from build123d import *
from build123d.topology import SkipClean

# Parameters (mm, degrees)
BOSS_EXTRUDE1_DEPTH     = 2
SKETCH2_R               = 1.9
BOSS_EXTRUDE2_DEPTH     = 2
CUT_EXTRUDE1_REACH      = 24.481
SKETCH4_R               = 4
BOSS_EXTRUDE3_REACH     = 24.481
BOSS_EXTRUDE4_DEPTH     = 2
BOSS_EXTRUDE5_DEPTH     = 2
CUT_EXTRUDE2_DEPTH      = 0.3
REVOLVE1_ANGLE          = 180
CUT_EXTRUDE3_DEPTH      = 24.576202563
CUT_EXTRUDE3_DEPTH_BACK = 24.576202563


with BuildPart() as part:
    # Sketch1 → Boss-Extrude1 (new body)
    with BuildSketch(Plane.XY):
        with BuildLine():
            Line((-4, -10), (4, -10))
            ThreePointArc((4, -10), (5.414213562, -9.414213562), (6, -8))
            Line((6, -8), (6, 6))
            Line((6, 6), (3.305891799, 20.36857707))
            ThreePointArc((3.305891799, 20.36857707), (2.6174191, 21.539018216), (1.340147425, 22))
            Line((1.340147425, 22), (-1.340147425, 22))
            ThreePointArc((-1.340147425, 22), (-2.6174191, 21.539018216), (-3.305891799, 20.36857707))
            Line((-3.305891799, 20.36857707), (-6, 6))
            Line((-6, 6), (-6, -8))
            ThreePointArc((-6, -8), (-5.414213562, -9.414213562), (-4, -10))
        make_face()
    extrude(amount=BOSS_EXTRUDE1_DEPTH)

    # Sketch2 → Boss-Extrude2 (add)
    with BuildSketch(Plane(origin=(0, 1.005401315, 5.701914197), x_dir=(-1, 0, 0), z_dir=(0, 0.1736481776669307, 0.984807753012208))):
        with BuildLine():
            Line((-3.6, -1.961550163), (-3.6, -5.561550163))
            Line((-3.6, -5.561550163), (-6, -5.561550163))
            Line((-6, -5.561550163), (-3.305891799, -19.711836261))
            add(Edge.make_bspline(
                [(-3.305891799, -19.711836261), (-3, -21.318474211), (-1.340147425, -21.318474211)],
                knots=[3.326940604, 3.326940604, 3.326940604, 4.71238898, 4.71238898, 4.71238898], degree=2, weights=[1, 0.769509108, 1]))
            Line((-1.340147425, -21.318474211), (1.340147425, -21.318474211))
            add(Edge.make_bspline(
                [(1.340147425, -21.318474211), (3, -21.318474211), (3.305891799, -19.711836261)],
                knots=[4.71238898, 4.71238898, 4.71238898, 6.097837357, 6.097837357, 6.097837357], degree=2, weights=[1, 0.769509108, 1]))
            Line((3.305891799, -19.711836261), (6, -5.561550163))
            Line((6, -5.561550163), (3.6, -5.561550163))
            Line((3.6, -5.561550163), (3.6, -1.961550163))
            ThreePointArc((3.6, -1.961550163), (0, 1.638449837), (-3.6, -1.961550163))
        make_face()
        with Locations(Location((0, -1.961550163, 0), (0, 0, 90))):
            Circle(SKETCH2_R, mode=Mode.SUBTRACT)
    extrude(amount=-BOSS_EXTRUDE2_DEPTH)

    # Cut-Extrude1: up to this plane
    cut_extrude1_end = Plane(origin=(1.340147425, 20, 0), z_dir=(0, 0, 1))
    # Sketch4 → Cut-Extrude1 (cut, up to the surface)
    with BuildSketch(Plane(origin=(0, 0.658104959, 3.732298691), x_dir=(-1, 0, 0), z_dir=(0, -0.1736481776669307, -0.9848077530122081)), mode=Mode.PRIVATE) as cut_extrude1_sk1:
        with Locations(Location((0, 1.961550163, 0), (0, 0, 90))):
            Circle(SKETCH4_R)
    cut_extrude1_tool1 = split(extrude(cut_extrude1_sk1.sketch, amount=CUT_EXTRUDE1_REACH, mode=Mode.PRIVATE), bisect_by=cut_extrude1_end, keep=Keep.BOTH, mode=Mode.PRIVATE)
    add(cut_extrude1_tool1.solids().sort_by_distance((0, 2.589855, 3.391679))[0], mode=Mode.SUBTRACT)

    # Sketch5 → Boss-Extrude3 (add, up to next)
    with BuildSketch(Plane(origin=(0, 0.658104959, 3.732298691), x_dir=(-1, 0, 0), z_dir=(0, -0.1736481776669307, -0.9848077530122081)), mode=Mode.PRIVATE) as boss_extrude3_sk1:
        with BuildLine():
            Line((-6, 5.561550163), (-4, 5.561550163))
            ThreePointArc((-4, 5.561550163), (0, 7.342999782), (4, 5.561550163))
            Line((4, 5.561550163), (6, 5.561550163))
            Line((6, 5.561550163), (5.159538931, 9.975910572))
            Line((5.159538931, 9.975910572), (-5.159538931, 9.975910572))
            Line((-5.159538931, 9.975910572), (-6, 5.561550163))
        make_face()
    boss_extrude3_tool1 = extrude(boss_extrude3_sk1.sketch, amount=BOSS_EXTRUDE3_REACH, mode=Mode.PRIVATE) - part.part
    add(boss_extrude3_tool1.solids().sort_by_distance((0, 8.606511, 2.33078))[0])

    # Sketch6 → Boss-Extrude4 (add)
    with BuildSketch(Plane(origin=(6, 0, 0), x_dir=(0, 0, -1), z_dir=(1, 0, 0))):
        Polygon((-4.736161147, 6.482459034), (-2, 6), (-2, -8), align=None)
    extrude(amount=-BOSS_EXTRUDE4_DEPTH)

    # Sketch7 → Boss-Extrude5 (add)
    with BuildSketch(Plane.ZY.offset(6)):
        Polygon((2, 6), (4.736161147, 6.482459034), (2, -8), align=None)
    extrude(amount=-BOSS_EXTRUDE5_DEPTH)

    # Sketch8 → Cut-Extrude2 (cut)
    with BuildSketch(Plane(origin=(0, 0, 0), x_dir=(-1, 0, 0), z_dir=(0, 0, -1))):
        with BuildLine():
            Line((-4, -3.5), (4, -3.5))
            ThreePointArc((4, -3.5), (4.75, -4.25), (4, -5))
            Line((4, -5), (-4, -5))
            ThreePointArc((-4, -5), (-4.75, -4.25), (-4, -3.5))
        make_face()
        with BuildLine():
            Line((-4, -6.5), (4, -6.5))
            ThreePointArc((4, -6.5), (4.75, -7.25), (4, -8))
            Line((4, -8), (-4, -8))
            ThreePointArc((-4, -8), (-4.75, -7.25), (-4, -6.5))
        make_face()
    extrude(amount=-CUT_EXTRUDE2_DEPTH, mode=Mode.SUBTRACT)

    # Sketch9 → Revolve1 (revolve)
    with BuildSketch(Plane(origin=(0, 1.005401315, 5.701914197), x_dir=(1, 0, 0), z_dir=(0, 0.1736481776669307, 0.9848077530122081))):
        with BuildLine():
            Line((-2, 16.318474211), (2, 16.318474211))
            ThreePointArc((2, 16.318474211), (0, 14.318474211), (-2, 16.318474211))
        make_face()
    revolve(axis=Axis((0, 17.075961235, 2.868240888), (-1, 0, 0)), revolution_arc=REVOLVE1_ANGLE)

    # Sketch11 → Cut-Extrude3 (cut, two sides)
    with SkipClean():  # the faces are left unmerged after this step: merging them gives an invalid solid
        with BuildSketch(Plane(origin=(0, 0, 0), x_dir=(0, 0, -1), z_dir=(1, 0, 0))) as cut_extrude3_sk:
            Polygon((-4.868240888, 17.075961235), (-2.868240888, 19.075961235), (-5.75514434, 19.075961235), align=None)
        extrude(amount=CUT_EXTRUDE3_DEPTH, mode=Mode.SUBTRACT)
        extrude(cut_extrude3_sk.sketch, amount=-CUT_EXTRUDE3_DEPTH_BACK, mode=Mode.SUBTRACT)


solid = part.part
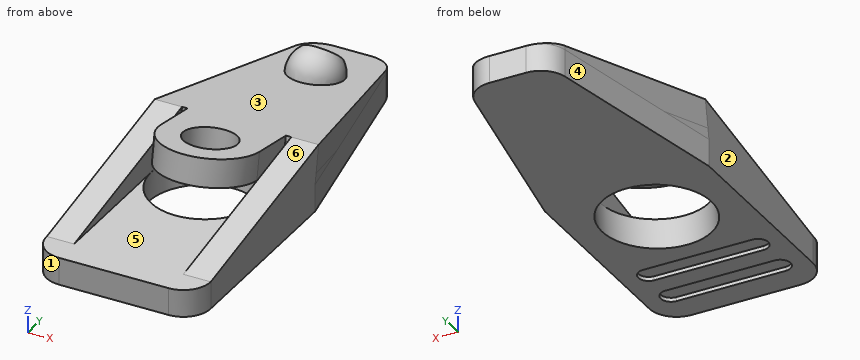
Verification items for the finished model (mm, model axes). Face numbers are marked on the shaded views. A direction names the side the tool comes from. Coordinates: 2 decimals unless noted, no trailing zeros. Order: outer loops, then holes, each group sorted by start corner. A loop starts at its lowest first (then second) coordinate and runs counter-clockwise, first axis right, second up. Notation, with made-up numbers: (-22, 63) -> (14, 63) arc R34 ccw to (14, 95) -> close; hole circle Ø9 at (7, 56). An arc over 180 degrees is marked (long way). Put each result on its own line as item: value. Start each with the question number.
1. Cross-section at B-B, the plane y = 13. Record the boundary of the cut face in (x, z), then the cut area to 3 significant figures.
2. Mould release check, pull along Y, two halves, no side actions. Record for the marked faces 1, 2 and 3: released by +Y, released by -Y, zero draft, split by the parting line, or undercut.
3. Go/stop test with flat-tipped pins: pin 1 Ø0.8 at (x, y) = (1, -7) entering from -Z; pin 2 Ø1 at (x, z) = (3, 2.5) entering from +Y; pin 3 Ø2 at (x, z) = (0, 4.5) entering from +Y; pin 4 Ø1.5 at (y, z) = (-3.5, 4.5) entering from -X. Record where each tip stops, or that it passes through.
4. Material ranges on L1, parallel to X at y = 2, z = 2.5; L2, parallel to Z at x = 2.5, y = -2.5; L3, parallel to X at y = 5, z = 1.45, recorded low to high. Write a range as [from, to].
5. Cross-section at A-A, the plane y = -4.25. Record the boundary of the cut face in (x, z).
6. Access from +Z, -Z, +X, -X, +Y, -Y to the whole of each face (thin tool, end or side, straight path). Record for the marked faces 4, 5 and 6.
Computed:
1. outline: (-4.74, 3.59) -> (-4.69, 2) -> (-4.69, 0) -> (4.69, 0) -> (4.69, 2) -> (4.74, 3.59) -> close
1. area: 33.7 mm2
2. face 1: released by -Y
2. face 2: zero draft
2. face 3: undercut
3. pin 1: z = 0.3
3. pin 2: y = 21.47
3. pin 3: y = 18.44
3. pin 4: through
4. L1: [-6, -4], [4, 6]
4. L2: [0, 2]
4. L3: [-6, -2.94], [2.94, 6]
5. outline: (-6, 0) -> (-4.75, 0) -> (-4.75, 0.3) -> (4.75, 0.3) -> (4.75, 0) -> (6, 0) -> (6, 2.71) -> (4, 2.71) -> (4, 2) -> (-4, 2) -> (-4, 2.71) -> (-6, 2.71) -> close
6. face 4: -Z, -X, +Y
6. face 5: +Z, -Y
6. face 6: +Z, +X, -Y
